```python
from build123d import *

# Parameters (mm, degrees)
BOSS_EXTRUDE1_DEPTH = 18
SKETCH2_R           = 2.5
CUT_EXTRUDE1_DEPTH  = 4


with BuildPart() as part:
    # Sketch1 → Boss-Extrude1 (new body)
    with BuildSketch(Plane.XY):
        with BuildLine():
            Line((-15.5, -28), (15.5, -28))
            ThreePointArc((15.5, -28), (17.621320344, -27.121320344), (18.5, -25))
            Line((18.5, -25), (18.5, 25))
            ThreePointArc((18.5, 25), (17.621320344, 27.121320344), (15.5, 28))
            Line((15.5, 28), (-15.5, 28))
            ThreePointArc((-15.5, 28), (-17.621320344, 27.121320344), (-18.5, 25))
            Line((-18.5, 25), (-18.5, -25))
            ThreePointArc((-18.5, -25), (-17.621320344, -27.121320344), (-15.5, -28))
        make_face()
    extrude(amount=BOSS_EXTRUDE1_DEPTH)

    # Sketch2 → Cut-Extrude1 (cut)
    with BuildSketch(Plane.XY.offset(18)):
        with Locations((-9.5, 18)):
            Circle(SKETCH2_R)
        with Locations((-9.5, -18)):
            Circle(SKETCH2_R)
        with Locations(Location((9.5, -18, 0), (0, 0, 180))):
            Circle(SKETCH2_R)
        with Locations(Location((9.5, 18, 0), (0, 0, 180))):
            Circle(SKETCH2_R)
    extrude(amount=-CUT_EXTRUDE1_DEPTH, mode=Mode.SUBTRACT)


solid = part.part
```
Input: part model. Units: mm. Frame: model coordinates. A direction names the side the tool comes from. Give positions to 0.01 mm unless a question says otherwise; leave off trailing zeros. Order: outer loops, then holes, each group sorted by start corner. A loop starts at its lowest first (then second) coordinate and runs counter-clockwise, first axis right, second up. Notation, with made-up numbers: (55, 70.5) -> (108, 70.5) arc R28 ccw to (108, 97.5) -> close; hole circle Ø3 at (42, 52.25). An arc over 180 degrees is marked (long way). Write each question's results on one line, items separated by ' | '. Start each with the question number.
Item 1: Cut plane C-C on x = 9.5. Return the cut outline in (y, z).
Item 2: Mould query, pull axis Y, two halves, no side actions, for faces 1 (the cylindrical face through (9.83, -20.48, 16.03)), 2 (the flat face through (0, 0, 18)), 3 (the cylindrical face through (-17.64, -27.1, 8.87)). Classes: pulls with the +Y half, pulls with the -Y half, needs draft (parallel to the pull), parting line crosses it, or undercut.
Item 3: Cut plane B-B on z = 14.75. Return the cut outline in (x, y).
Item 4: Set-up query: faces 4 (the flat face through (-10, 18, 14)), 5 (the cylindrical face through (-17.6, 27.14, 8.87)). Return all of +Z, -Z, +X, -X, +Y, -Y with unobstructed straight access to the full face (end or side cutting, diameter ignored); none if empty.
Item 5: Contact query for a flat-ended pin moving along its axis: P1, Ø4.5, axis at x = 9.5, y = -18, coming from the +Z side. Output: stop coordinate, or through.
Item 6: Cut plane A-A on y = -18. Return the cut outline in (x, z), then the cut area to 3 significant figures.
Item 7: Line query: line 1 (Y direction, x = 9.5, z = 15.5); line 2 (X direction, y = -20, z = 14.75); line 3 (Y direction, x = 10, z = 16.5). Output: solid intervals per line, ascending.
Established:
1) outline: (-28, 0) -> (28, 0) -> (28, 18) -> (20.5, 18) -> (20.5, 14) -> (15.5, 14) -> (15.5, 18) -> (-15.5, 18) -> (-15.5, 14) -> (-20.5, 14) -> (-20.5, 18) -> (-28, 18) -> close
2) face 1: undercut | face 2: needs draft | face 3: pulls with the -Y half
3) outline: (-18.5, -25) arc R3 ccw to (-15.5, -28) -> (15.5, -28) arc R3 ccw to (18.5, -25) -> (18.5, 25) arc R3 ccw to (15.5, 28) -> (-15.5, 28) arc R3 ccw to (-18.5, 25) -> close; hole circle Ø5 at (-9.5, -18); hole circle Ø5 at (-9.5, 18); hole circle Ø5 at (9.5, -18); hole circle Ø5 at (9.5, 18)
4) face 4: +Z | face 5: +Z, -Z, -X, +Y
5) P1: z = 14
6) outline: (-18.5, 0) -> (18.5, 0) -> (18.5, 18) -> (12, 18) -> (12, 14) -> (7, 14) -> (7, 18) -> (-7, 18) -> (-7, 14) -> (-12, 14) -> (-12, 18) -> (-18.5, 18) -> close | area: 626 mm^2
7) line 1: -28 to -20.5, -15.5 to 15.5, 20.5 to 28 | line 2: -18.5 to -11, -8 to 8, 11 to 18.5 | line 3: -28 to -20.45, -15.55 to 15.55, 20.45 to 28
